Part model, mm, in its own coordinate system. Face numbers are marked on the shaded views. A direction names the side the tool comes from. Give positions to 0.01 mm unless a question says otherwise; leave off trailing zeros. Write each loop counter-clockwise with the first axis right and the second up, starting at its lowest first coordinate (ties: lowest second). Pieces come first, ordered by that corner, then holes.
```python
from build123d import *

# Parameters (mm, degrees)
CROQUIS1_W              = 37.5
CROQUIS1_H              = 30
SALIENTE_EXTRUIR1_DEPTH = 15
CROQUIS2_R              = 4
SALIENTE_EXTRUIR2_DEPTH = 8
SALIENTE_EXTRUIR3_DEPTH = 35
CROQUIS5_W              = 18
CROQUIS5_H              = 12
CROQUIS5_R              = 4.5
SALIENTE_EXTRUIR4_DEPTH = 5
CROQUIS6_W              = 1
CROQUIS6_H              = 12
CORTAR_EXTRUIR2_DEPTH   = 14
CROQUIS7_W              = 58.738074731
CROQUIS7_H              = 36.211204921
CORTAR_EXTRUIR4_DEPTH   = 75.820201149
CORTAR_EXTRUIR5_DEPTH   = 30
SALIENTE_EXTRUIR5_DEPTH = 100


with BuildPart() as part:
    # Croquis1 → Saliente-Extruir1 (new body)
    with BuildSketch(Plane.XY):
        Rectangle(CROQUIS1_W, CROQUIS1_H)
    extrude(amount=SALIENTE_EXTRUIR1_DEPTH)

    # Croquis2 → Saliente-Extruir2 (add)
    with BuildSketch(Plane.XY):
        with BuildLine():
            Line((-18.75, 6), (-29.75, 6))
            ThreePointArc((-29.75, 6), (-30.457106781, 5.707106781), (-30.75, 5))
            Line((-30.75, 5), (-30.75, -5))
            ThreePointArc((-30.75, -5), (-30.457106781, -5.707106781), (-29.75, -6))
            Line((-29.75, -6), (-18.75, -6))
            Line((-18.75, -6), (-18.75, 6))
        make_face()
        with Locations((-24.75, 0)):
            Circle(CROQUIS2_R, mode=Mode.SUBTRACT)
    extrude(amount=SALIENTE_EXTRUIR2_DEPTH)

    # Croquis3 → Saliente-Extruir3 (add)
    with BuildSketch(Plane(origin=(18.75, 0, 0), x_dir=(0, 0, -1), z_dir=(1, 0, 0))):
        with BuildLine():
            Line((-10.5, -12.5), (-4.5, -12.5))
            ThreePointArc((-4.5, -12.5), (-2.378679656, -11.621320344), (-1.5, -9.5))
            Line((-1.5, -9.5), (-1.5, 9.5))
            ThreePointArc((-1.5, 9.5), (-2.378679656, 11.621320344), (-4.5, 12.5))
            Line((-4.5, 12.5), (-10.5, 12.5))
            ThreePointArc((-10.5, 12.5), (-12.621320344, 11.621320344), (-13.5, 9.5))
            Line((-13.5, 9.5), (-13.5, -9.5))
            ThreePointArc((-13.5, -9.5), (-12.621320344, -11.621320344), (-10.5, -12.5))
        make_face()
    extrude(amount=SALIENTE_EXTRUIR3_DEPTH)

    # Croquis5 → Saliente-Extruir4 (add, symmetric)
    with BuildSketch(Plane.XY.offset(7.5)):
        with Locations((62.75, 0)):
            Rectangle(CROQUIS5_W, CROQUIS5_H)
        with Locations((62.75, 0)):
            Circle(CROQUIS5_R, mode=Mode.SUBTRACT)
    extrude(amount=SALIENTE_EXTRUIR4_DEPTH, both=True)

    # Croquis6 → Cortar-Extruir2 (cut)
    with BuildSketch(Plane(origin=(71.75, 0, 0), x_dir=(0, 0, -1), z_dir=(1, 0, 0))):
        with Locations((-12, 0)):
            Rectangle(CROQUIS6_W, CROQUIS6_H)
        with Locations((-3, 0)):
            Rectangle(CROQUIS6_W, CROQUIS6_H)
    extrude(amount=-CORTAR_EXTRUIR2_DEPTH, mode=Mode.SUBTRACT)

    # Croquis7 → Cortar-Extruir4 (cut, through all)
    with BuildSketch(Plane.XY.offset(15)):
        with Locations((83.119037366, -6.200481031)):
            Rectangle(CROQUIS7_W, CROQUIS7_H)
    extrude(amount=-CORTAR_EXTRUIR4_DEPTH, mode=Mode.SUBTRACT)

    # Croquis8 → Cortar-Extruir5 (cut)
    with BuildSketch(Plane(origin=(53.75, 0, 0), x_dir=(0, 0, -1), z_dir=(1, 0, 0))):
        with BuildLine():
            Line((-9.5, -6), (-5.5, -6))
            ThreePointArc((-5.5, -6), (-3.378679656, -5.121320344), (-2.5, -3))
            Line((-2.5, -3), (-2.5, 3))
            ThreePointArc((-2.5, 3), (-3.378679656, 5.121320344), (-5.5, 6))
            Line((-5.5, 6), (-9.5, 6))
            ThreePointArc((-9.5, 6), (-11.621320344, 5.121320344), (-12.5, 3))
            Line((-12.5, 3), (-12.5, -3))
            ThreePointArc((-12.5, -3), (-11.621320344, -5.121320344), (-9.5, -6))
        make_face()
    extrude(amount=-CORTAR_EXTRUIR5_DEPTH, mode=Mode.SUBTRACT)

    # Croquis10 → Saliente-Extruir5 (add)
    with BuildSketch(Plane(origin=(53.75, 0, 0), x_dir=(0, 0, -1), z_dir=(1, 0, 0))):
        with BuildLine():
            Line((-13.5, 9.5), (-13.5, -9.5))
            ThreePointArc((-13.5, -9.5), (-12.621320344, -11.621320344), (-10.5, -12.5))
            Line((-10.5, -12.5), (-4.5, -12.5))
            ThreePointArc((-4.5, -12.5), (-2.378679656, -11.621320344), (-1.5, -9.5))
            Line((-1.5, -9.5), (-1.5, 9.5))
            ThreePointArc((-1.5, 9.5), (-2.378679656, 11.621320344), (-4.5, 12.5))
            Line((-4.5, 12.5), (-10.5, 12.5))
            ThreePointArc((-10.5, 12.5), (-12.621320344, 11.621320344), (-13.5, 9.5))
        make_face()
        with BuildLine():
            Line((-2.5, -3), (-2.5, 3))
            ThreePointArc((-2.5, 3), (-3.378679656, 5.121320344), (-5.5, 6))
            Line((-5.5, 6), (-9.5, 6))
            ThreePointArc((-9.5, 6), (-11.621320344, 5.121320344), (-12.5, 3))
            Line((-12.5, 3), (-12.5, -3))
            ThreePointArc((-12.5, -3), (-11.621320344, -5.121320344), (-9.5, -6))
            Line((-9.5, -6), (-5.5, -6))
            ThreePointArc((-5.5, -6), (-3.378679656, -5.121320344), (-2.5, -3))
        make_face(mode=Mode.SUBTRACT)
    extrude(amount=SALIENTE_EXTRUIR5_DEPTH)


solid = part.part
```
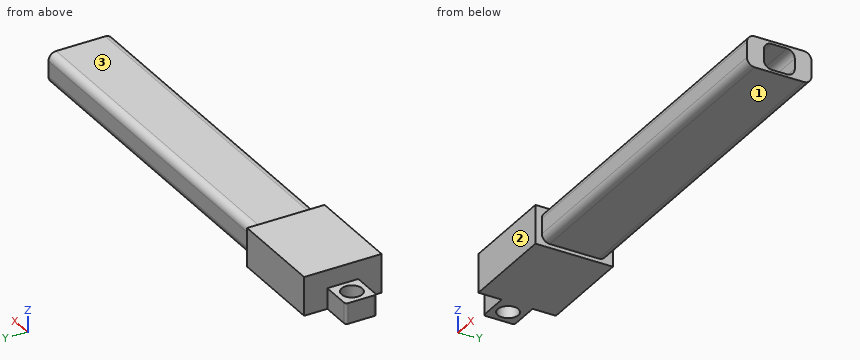
1) Saw through at D-D, the plane x = 21. Write the cut outline in (y, z), then the cut area to 3 significant figures.
Answers follow:
outline: (-12.5, 4.5) arc R3 ccw to (-9.5, 1.5) - (9.5, 1.5) arc R3 ccw to (12.5, 4.5) - (12.5, 10.5) arc R3 ccw to (9.5, 13.5) - (-9.5, 13.5) arc R3 ccw to (-12.5, 10.5) - close
area: 292 mm2
2) Saw through at A-A, the plane y = 0. Write the cut outline in (x, z).
Answers follow:
outline: (-30.75, 0) - (-28.75, 0) - (-28.75, 8) - (-30.75, 8) - close; (-20.75, 0) - (18.75, 0) - (18.75, 1.5) - (153.75, 1.5) - (153.75, 2.5) - (23.75, 2.5) - (23.75, 12.5) - (153.75, 12.5) - (153.75, 13.5) - (18.75, 13.5) - (18.75, 15) - (-18.75, 15) - (-18.75, 8) - (-20.75, 8) - close
3) Saw through at B-B, the plane x = 113. Write the cut outline in (y, z).
Answers follow:
outline: (-12.5, 4.5) arc R3 ccw to (-9.5, 1.5) - (9.5, 1.5) arc R3 ccw to (12.5, 4.5) - (12.5, 10.5) arc R3 ccw to (9.5, 13.5) - (-9.5, 13.5) arc R3 ccw to (-12.5, 10.5) - close; hole (-6, 5.5) arc R3 ccw to (-3, 2.5) - (3, 2.5) arc R3 ccw to (6, 5.5) - (6, 9.5) arc R3 ccw to (3, 12.5) - (-3, 12.5) arc R3 ccw to (-6, 9.5) - close
4) 3-axis set-ups, long thin cutter, end or side, ignore diameter. For the marked faces 1, 2 and 3: which of +Z, -Z, +X, -X, +Y, -Y reach the whole face in a straight line?
Answers follow:
face 1: -Z, +X, +Y, -Y
face 2: +Z, -Z, +X, -X, -Y
face 3: +Z, +X, +Y, -Y
5) Wall check: L1, parallel to Y at x = -24.75, z = 4.5; L2, parallel to Y at x = 84.5, z = 8.5; L3, parallel to Z at x = 53, y = 0.5. Give the ranges that are in metal, low to high.
Answers follow:
L1: y = -6 to -4, 4 to 6
L2: y = -12.5 to -6, 6 to 12.5
L3: z = 1.5 to 2.5, 12.5 to 13.5
6) Saw through at C-C, the plane x = -24.75. Write the cut outline in (y, z), then the cut area to 3 significant figures.
Answers follow:
outline: (-6, 0) - (-4, 0) - (-4, 8) - (-6, 8) - close; (4, 0) - (6, 0) - (6, 8) - (4, 8) - close
area: 32.0 mm2
7) Pin check, flat tips, straight feed: pin 1 Ø1.8 at (x, y) = (93.5, -1) entering from -Z; pin 2 Ø3.5 at (x, y) = (-25, -1) entering from +Z; pin 3 Ø4.5 at (x, z) = (69.5, 8.5) entering from -Y; pin 4 Ø3 at (x, z) = (104.5, 6.5) entering from +Y. Stop position of each tip, or through.
Answers follow:
pin 1: stops at z = 1.5
pin 2: passes through
pin 3: stops at y = -12.5
pin 4: stops at y = 12.5
